from build123d import *

# Parameters (mm, degrees)
EXTRUDE_1_DEPTH     = 5
SKETCH_2_W          = 30
SKETCH_2_H          = 30
SKETCH_2_H_2        = 25
CUT_EXTRUDE_1_DEPTH = 189.903823128
CHAMFER_1_SIZE      = 4
EXTRUDE_2_DEPTH     = 15
CUT_EXTRUDE_2_DEPTH = 3
CUT_EXTRUDE_3_DEPTH = 3
CUT_EXTRUDE_4_DEPTH = 3
CUT_EXTRUDE_5_DEPTH = 3
FILLET_1_R          = 3
SKETCH_8_W          = 91.7
SKETCH_8_H          = 142
CUT_EXTRUDE_6_DEPTH = 5


with BuildPart() as part:
    # 草图1 → 凸台-拉伸1 (new body)
    with BuildSketch(Plane.XY):
        with BuildLine():
            Line((-45, 115), (-45, 120))
            ThreePointArc((-45, 120), (-42.071067812, 127.071067812), (-35, 130))
            Line((-35, 130), (35.124730195, 130))
            ThreePointArc((35.124730195, 130), (42.10760044, 127.10760044), (45, 120.124730195))
            Line((45, 120.124730195), (45, 115))
            ThreePointArc((45, 115), (47.928932188, 107.928932188), (55, 105))
            Line((55, 105), (126, 105))
            ThreePointArc((126, 105), (133.071067812, 102.071067812), (136, 95))
            Line((136, 95), (136, -95))
            ThreePointArc((136, -95), (133.071067812, -102.071067812), (126, -105))
            Line((126, -105), (115, -105))
            Line((115, -105), (55, -105))
            ThreePointArc((55, -105), (47.928932188, -107.928932188), (45, -115))
            Line((45, -115), (45, -121.010130877))
            ThreePointArc((45, -121.010130877), (42.071067812, -128.081198689), (35, -131.010130877))
            Line((35, -131.010130877), (-35, -131.010130877))
            ThreePointArc((-35, -131.010130877), (-42.071067812, -128.081198689), (-45, -121.010130877))
            Line((-45, -121.010130877), (-45, -115))
            ThreePointArc((-45, -115), (-47.928932188, -107.928932188), (-55, -105))
            Line((-55, -105), (-114, -105))
            Line((-114, -105), (-114, -95))
            Line((-114, -95), (-114, 95))
            Line((-114, 95), (-114, 105))
            Line((-114, 105), (-55, 105))
            ThreePointArc((-55, 105), (-47.928932188, 107.928932188), (-45, 115))
        make_face()
    extrude(amount=EXTRUDE_1_DEPTH)

    # 草图2 → 切除-拉伸1 (cut, through all)
    with BuildSketch(Plane.XY.offset(5)):
        with Locations((-81, 82)):
            Rectangle(SKETCH_2_W, SKETCH_2_H)
        with Locations((-81, -82)):
            Rectangle(SKETCH_2_W, SKETCH_2_H)
        with Locations((103, 82)):
            Rectangle(SKETCH_2_W, SKETCH_2_H_2)
        with Locations((103, -82)):
            Rectangle(SKETCH_2_W, SKETCH_2_H_2)
        Polygon((3, 94.5), (63, 94.5), (63, 69.5), align=None)
        Polygon((3, -94.5), (63, -94.5), (63, -69.5), align=None)
    extrude(amount=-CUT_EXTRUDE_1_DEPTH, mode=Mode.SUBTRACT)

    # 倒角1
    chamfer_1_edges = [part.edges().sort_by_distance(p)[0] for p in [
        (118, -69.5, 2.5),
        (118, -94.5, 2.5),
        (88, -94.5, 2.5),
        (88, -69.5, 2.5),
        (118, 94.5, 2.5),
        (118, 69.5, 2.5),
        (88, 69.5, 2.5),
        (88, 94.5, 2.5),
        (-66, -67, 2.5),
        (-66, -97, 2.5),
        (-96, -97, 2.5),
        (-96, -67, 2.5),
        (-66, 97, 2.5),
        (-66, 67, 2.5),
        (-96, 67, 2.5),
        (-96, 97, 2.5),
    ]]
    chamfer(chamfer_1_edges, length=CHAMFER_1_SIZE)

    # 草图3 → 凸台-拉伸2 (add)
    with BuildSketch(Plane(origin=(0, 0, 0), x_dir=(-1, 0, 0), z_dir=(0, 0, -1))):
        Polygon((-131, 66), (-131, 55), (-128, 55), (-128, 63), (-120, 63), (-120, 66), align=None)
        Polygon((-56, 63), (-56, 66), (-45, 66), (-45, 55), (-48, 55), (-48, 63), align=None)
        Polygon((-48, -63), (-56, -63), (-56, -66), (-45, -66), (-45, -55), (-48, -55), align=None)
        Polygon((-120, -63), (-120, -66), (-131, -66), (-131, -55), (-128, -55), (-128, -63), align=None)
    extrude(amount=EXTRUDE_2_DEPTH)

    # 草图4 → 切除-拉伸2 (cut)
    with BuildSketch(Plane(origin=(131, 0, 0), x_dir=(0, 0, -1), z_dir=(1, 0, 0))):
        Polygon((15, 60.5), (5, 55), (15, 55), align=None)
        Polygon((15, -60.5), (15, -55), (5, -55), align=None)
    extrude(amount=-CUT_EXTRUDE_2_DEPTH, mode=Mode.SUBTRACT)

    # 草图5 → 切除-拉伸3 (cut)
    with BuildSketch(Plane(origin=(0, 66, 0), x_dir=(1, 0, 0), z_dir=(0, 1, 0))):
        Polygon((50.5, 15), (56, 15), (56, 5), align=None)
        Polygon((120, 15), (125.5, 15), (120, 5), align=None)
    extrude(amount=-CUT_EXTRUDE_3_DEPTH, mode=Mode.SUBTRACT)

    # 草图6 → 切除-拉伸4 (cut)
    with BuildSketch(Plane.ZY.offset(-45)):
        Polygon((-15, 60.5), (-5, 55), (-15, 55), align=None)
        Polygon((-15, -60.5), (-15, -55), (-5, -55), align=None)
    extrude(amount=-CUT_EXTRUDE_4_DEPTH, mode=Mode.SUBTRACT)

    # 草图7 → 切除-拉伸5 (cut)
    with BuildSketch(Plane.XZ.offset(66)):
        Polygon((50.5, -15), (56, -15), (56, -5), align=None)
        Polygon((120, -15), (125.5, -15), (120, -5), align=None)
    extrude(amount=-CUT_EXTRUDE_5_DEPTH, mode=Mode.SUBTRACT)

    # 圆角1
    fillet_1_edges = [part.edges().sort_by_distance(p)[0] for p in [
        (63, -69.5, 2.5),
        (63, -94.5, 2.5),
        (3, -94.5, 2.5),
        (63, 69.5, 2.5),
        (3, 94.5, 2.5),
        (63, 94.5, 2.5),
    ]]
    fillet(fillet_1_edges, radius=FILLET_1_R)

    # 草图8 → 切除-拉伸6 (cut)
    with BuildSketch(Plane(origin=(0, 0, 0), x_dir=(-1, 0, 0), z_dir=(0, 0, -1))):
        with Locations((3.85, 0)):
            Rectangle(SKETCH_8_W, SKETCH_8_H)
    extrude(amount=-CUT_EXTRUDE_6_DEPTH, mode=Mode.SUBTRACT)


solid = part.part
Here's how the part is built. I have some questions about the finished solid (model axes, mm). A direction names the side the tool comes from. Round coordinates to 2 decimals unless told otherwise and drop trailing zeros. Loops run counter-clockwise (first coordinate to the right, second up) from the corner with the lowest first, then second, coordinate; pieces in that order, holes last. Notation, with made-up numbers: M 38.25,-11 L 48.25,-11 A37 ccw 48.25,28 Z; hole C 26,-6 d8. An arc over 180 degrees is marked long. Write each question's results on one line, items separated by ' | '. Start each with the question number.
(1) Will these pins go through, and if not, where does the flat tip stop? P1, Ø1.5, axis at y = 64.5, z = -1.5, coming from the -X side; P2, Ø1.5, axis at x = -91.5, z = 3, coming from the +Y side; P3, Ø3.5, axis at x = 124, z = -9, coming from the -Y side; P4, Ø8, axis at y = 88, z = -4.5, coming from the -X side.
(2) If I drill on probe 1 along X at (y, z) = (5, 3.5); probe 2 along X at (y, z) = (60, -10); probe 3 along Z at (x, y) = (122, 74.5), over which ranges is the centre line in solid material (lowest first)? Write a range as from..to.
(3) I want a section at B-B (x = -2). Please give me the cut outline in (y, z).
(4) I want a section at A-A (y = 30). Please give me the cut outline in (x, z), then the cut area to 4 significant figures.
(5) I want a section at C-C (z = -9.5). Please give me the cut outline in (x, y) (3 decimals), then the cut area to 3 significant figures.
(6) I want a section at D-D (x = -74.5). Please give me the cut outline in (y, z).
(7) On a 3-axis mill with a long thin cutter (end or side, diameter ignored), from which of +Z, -Z, +X, -X, +Y, -Y can I reach the whole of each face in a straight line? I mean faces 4 (the flat face through (45, -62, -7)), 5 (the flat face through (49, 66, -7)), 6 (the flat face through (122.79, 64.52, -10.07)), 7 (the flat face through (48, -60, -6)), 8 (the flat face through (129.52, 57.79, -10.07)). Say none if no direction works.
(8) Thinking about a two-plate mould opening in Y: for faces 1 (the flat face through (129, 64, -15)), 2 (the flat face through (38.14, 79.86, 2.54)), 3 (the cylindrical face through (132.99, 102.15, 2.46)), which applies, pulls with the +Y half, pulls with the -Y half, needs draft (parallel to the pull), parting line crosses it, or undercut?
Solved:
1) P1: stops at x = 45 | P2: stops at y = 105 | P3: stops at y = -66 | P4: passes through
2) probe 1: x = -114..-49.7, 42..136 | probe 2: x = 45..48, 128..131 | probe 3: z = 0..5
3) outline: M -131.01,0 L -71,0 L -71,5 L -131.01,5 Z; M 71,0 L 130,0 L 130,5 L 71,5 Z
4) outline: M -114,0 L -49.7,0 L -49.7,5 L -114,5 Z; M 42,0 L 136,0 L 136,5 L 42,5 Z | area: 791.5 mm²
5) outline: M 45,-66 L 53.525,-66 L 53.525,-63 L 48,-63 L 48,-57.475 L 45,-57.475 Z; M 45,57.475 L 48,57.475 L 48,63 L 53.525,63 L 53.525,66 L 45,66 Z; M 122.475,-66 L 131,-66 L 131,-57.475 L 128,-57.475 L 128,-63 L 122.475,-63 Z; M 122.475,63 L 128,63 L 128,57.475 L 131,57.475 L 131,66 L 122.475,66 Z | area: 169 mm²
6) outline: M -105,0 L -97,0 L -97,5 L -105,5 Z; M -67,0 L 67,0 L 67,5 L -67,5 Z; M 97,0 L 105,0 L 105,5 L 97,5 Z
7) face 4: -Z, -X, +Y, -Y | face 5: -Z, +X, -X, +Y | face 6: -Z, +Y, -Y | face 7: -Z | face 8: -Z, +X, -X
8) face 1: needs draft | face 2: undercut | face 3: pulls with the +Y half
